Could you check a few things on this model? Use its own coordinates, in mm. A direction names the side the tool comes from. Round coordinates to 2 decimals unless told otherwise and drop trailing zeros. Order: outer loops, then holes, each group sorted by start corner. A loop starts at its lowest first (then second) coordinate and runs counter-clockwise, first axis right, second up. Notation, with made-up numbers: (12, 21) - (56, 21) arc R9 ccw to (56, 33) - close; hole circle Ø2 at (-8.75, -16). An arc over 180 degrees is marked (long way). Use one line per item in the form item = value.
from build123d import *

# Parameters (mm, degrees)
SKETCH1_R            = 63
BOSS_EXTRUDE4_DEPTH  = 4
SKETCH2_R            = 55
BOSS_EXTRUDE5_DEPTH  = 40
SKETCH3_R            = 51
CUT_EXTRUDE1_DEPTH   = 40
SKETCH9_W            = 40
SKETCH9_H            = 20
BOSS_EXTRUDE8_DEPTH  = 0.001
BOSS_EXTRUDE9_DEPTH  = 20
SKETCH12_R           = 1.5
CUT_EXTRUDE4_DEPTH   = 20
BOSS_EXTRUDE10_START = -9
SKETCH22_W           = 35
SKETCH22_H           = 35
BOSS_EXTRUDE10_DEPTH = 9
SKETCH24_W           = 32
SKETCH24_H           = 32
CUT_EXTRUDE15_DEPTH  = 7
FILLET6_R            = 1
SKETCH25_W           = 25
SKETCH25_H           = 17
CUT_EXTRUDE16_DEPTH  = 2
SKETCH26_R           = 1
CUT_EXTRUDE18_DEPTH  = 2
SKETCH30_W           = 12.5
SKETCH30_H           = 12.5
CUT_EXTRUDE24_DEPTH  = 3
SKETCH29_R           = 1.5
CUT_EXTRUDE25_DEPTH  = 4


with BuildPart() as part:
    # Sketch1 → Boss-Extrude4 (new body)
    with BuildSketch(Plane(origin=(0, 0, 0), x_dir=(1, 0, 0), z_dir=(0, 1, 0))):
        with Locations(Location((0, 0, 0), (0, 0, 270))):
            Circle(SKETCH1_R)
    extrude(amount=BOSS_EXTRUDE4_DEPTH)

    # Sketch2 → Boss-Extrude5 (add)
    with BuildSketch(Plane(origin=(0, 4, 0), x_dir=(1, 0, 0), z_dir=(0, 1, 0))):
        with Locations(Location((0, 0, 0), (0, 0, 270))):
            Circle(SKETCH2_R)
    extrude(amount=BOSS_EXTRUDE5_DEPTH)

    # Sketch3 → Cut-Extrude1 (cut)
    with BuildSketch(Plane.XZ):
        with Locations(Location((0, 0, 0), (0, 0, 270))):
            Circle(SKETCH3_R)
    extrude(amount=-CUT_EXTRUDE1_DEPTH, mode=Mode.SUBTRACT)

    # Sketch9 → Boss-Extrude8 (add)
    with BuildSketch(Plane(origin=(0, 44, 0), x_dir=(1, 0, 0), z_dir=(0, 1, 0))):
        Rectangle(SKETCH9_W, SKETCH9_H)
    extrude(amount=BOSS_EXTRUDE8_DEPTH)

    # Sketch11 → Boss-Extrude9 (add)
    with BuildSketch(Plane(origin=(0, 0, -10), x_dir=(-1, 0, 0), z_dir=(0, 0, -1))):
        with BuildLine():
            Line((-20, 44.001), (-20, 64.001))
            ThreePointArc((-20, 64.001), (0, 84.001), (20, 64.001))
            Line((20, 64.001), (20, 44.001))
            Line((20, 44.001), (-20, 44.001))
        make_face()
    extrude(amount=-BOSS_EXTRUDE9_DEPTH)

    # Sketch12 → Cut-Extrude4 (cut)
    with BuildSketch(Plane.XY.offset(10)):
        with Locations((0, 65)):
            Circle(SKETCH12_R)
    extrude(amount=-CUT_EXTRUDE4_DEPTH, mode=Mode.SUBTRACT)

    # Sketch22 → Boss-Extrude10 (add)
    with BuildSketch(Plane.XY.offset(55).offset(BOSS_EXTRUDE10_START)):
        with Locations((0, 23.97160628)):
            Rectangle(SKETCH22_W, SKETCH22_H)
    extrude(amount=BOSS_EXTRUDE10_DEPTH)

    # Sketch24 → Cut-Extrude15 (cut)
    with BuildSketch(Plane(origin=(0, 0, 46), x_dir=(-1, 0, 0), z_dir=(0, 0, -1))):
        with Locations((0, 23.722591491)):
            Rectangle(SKETCH24_W, SKETCH24_H)
    extrude(amount=-CUT_EXTRUDE15_DEPTH, mode=Mode.SUBTRACT)

    # Fillet6
    fillet6_edges = [part.edges().sort_by_distance(p)[0] for p in [
        (-20, 44, 0),
        (-20, 54.0005, -10),
        (0, 44, 10),
        (-20, 54.0005, 10),
        (20, 44, 0),
        (20, 54.0005, 10),
        (0, 44, -10),
        (20, 54.0005, -10),
        (0, 84.001, -10),
        (0, 84.001, 10),
    ]]
    fillet(fillet6_edges, radius=FILLET6_R)

    # Sketch25 → Cut-Extrude16 (cut)
    with BuildSketch(Plane.XY.offset(55)):
        with Locations((0, 24.10057748)):
            Rectangle(SKETCH25_W, SKETCH25_H)
    extrude(amount=-CUT_EXTRUDE16_DEPTH, mode=Mode.SUBTRACT)

    # Sketch26 → Cut-Extrude18 (cut)
    with BuildSketch(Plane.XY.offset(55)):
        with Locations((-11.5, 35.429004604)):
            Circle(SKETCH26_R)
        with Locations((11.5, 35.429004604)):
            Circle(SKETCH26_R)
        with Locations((11.5, 11.727594133)):
            Circle(SKETCH26_R)
        with Locations((-11.5, 11.727594133)):
            Circle(SKETCH26_R)
    extrude(amount=-CUT_EXTRUDE18_DEPTH, mode=Mode.SUBTRACT)

    # Sketch30 → Cut-Extrude24 (cut)
    with BuildSketch(Plane(origin=(0, 44, 0), x_dir=(1, 0, 0), z_dir=(0, 1, 0))):
        with Locations((20, -30)):
            Rectangle(SKETCH30_W, SKETCH30_H)
        with Locations((0, -30)):
            Rectangle(SKETCH30_W, SKETCH30_H)
        with Locations((-20, -30)):
            Rectangle(SKETCH30_W, SKETCH30_H)
    extrude(amount=-CUT_EXTRUDE24_DEPTH, mode=Mode.SUBTRACT)

    # Sketch29 → Cut-Extrude25 (cut)
    with BuildSketch(Plane(origin=(0, 4, 0), x_dir=(1, 0, 0), z_dir=(0, 1, 0))):
        with Locations(Location((0, 59, 0), (0, 0, 270))):
            Circle(SKETCH29_R)
        with Locations(Location((-50.985971771, -29.688898305, 0), (0, 0, 270))):
            Circle(SKETCH29_R)
        with Locations(Location((50.985971771, -29.688898305, 0), (0, 0, 270))):
            Circle(SKETCH29_R)
    extrude(amount=-CUT_EXTRUDE25_DEPTH, mode=Mode.SUBTRACT)


solid = part.part
Item 1: Imagine slicing it at A-A on z = 0. Please give me the cut outline in (x, y).
Found:
outline = (-63, 0) - (-51, 0) - (-51, 40) - (51, 40) - (51, 0) - (63, 0) - (63, 4) - (55, 4) - (55, 44) - (21, 44) arc R1 cw to (20, 45) - (20, 64) arc R20 ccw to (-20, 64) - (-20, 45) arc R1 cw to (-21, 44) - (-55, 44) - (-55, 4) - (-63, 4) - close; hole circle Ø3 at (0, 65)
Item 2: For faces 1 (the face through (0, 36, 55)), 2 (the face through (-20, 55, 0)), 3 (the face through (20, 43, 23.75)), 4 (the face through (-16, 23, 49)), which set-ups out of +Z, -Z, +X, -X, +Y, -Y let a thin tool reach every point of the face, with its end or its side?
Found:
face_1 = +Z, +X, -X, +Y
face_2 = +Z, -Z, -X, +Y
face_3 = +Y
face_4 = none
Item 3: Imagine slicing it at C-C on z = -48. Please give me the cut outline in (x, y), plus the area to 3 significant figures.
Found:
outline = (-40.8, 0) - (-17.23, 0) - (-17.23, 40) - (17.23, 40) - (17.23, 0) - (40.8, 0) - (40.8, 4) - (26.85, 4) - (26.85, 44) - (-26.85, 44) - (-26.85, 4) - (-40.8, 4) - close
area = 1,100 mm2
Item 4: Imagine slicing it at D-D on x = 38.5. Please give me the cut outline in (y, z).
Found:
outline = (0, -49.87) - (4, -49.87) - (4, -39.28) - (44, -39.28) - (44, 39.28) - (4, 39.28) - (4, 49.87) - (0, 49.87) - (0, 33.45) - (40, 33.45) - (40, -33.45) - (0, -33.45) - close
Item 5: Will these pins go through, and if not, where does the flat tip stop? P1, Ø1, axis at x = 1, y = 58.5, coming from the -Z side; P2, Ø3, axis at x = 11.5, y = 35.43, coming from the +Z side; P3, Ø2.5, axis at x = 17.5, y = 42, coming from the -Z side.
Found:
P1 = -10
P2 = 55
P3 = -52.54
Item 6: I need wall thicknesses on L1, parallel to Y at x = 11.5, z = 54.05; L2, parallel to X at y = 65, z = 3.75; L3, parallel to Y at x = 37, z = -1. Which ranges of each line are inside material? Lowest first, please.
Found:
L1 = 0 to 4, 6.47 to 10.73, 12.73 to 15.6, 32.6 to 34.43, 36.43 to 41.47
L2 = -19.98 to -1.5, 1.5 to 19.98
L3 = 40 to 44
Item 7: Imagine slicing it at B-B on y = 49. Please give me the cut outline in (x, z).
Found:
outline = (-20, -9) arc R1 ccw to (-19, -10) - (19, -10) arc R1 ccw to (20, -9) - (20, 9) arc R1 ccw to (19, 10) - (-19, 10) arc R1 ccw to (-20, 9) - close
Item 8: If we mould it in two halves opening along Y, with no side actions, what happens to faces 5 (the face through (16, 23, 49)), 6 (the face through (20, 54, 0)), 7 (the face through (0, 7.723, 49)), 8 (the face through (-51, 0, -5))? For each: released by +Y, released by -Y, zero draft, split by the parting line, or undercut.
Found:
face_5 = undercut
face_6 = zero draft
face_7 = undercut
face_8 = released by -Y
